from build123d import *

# Parameters (mm, degrees)
SKETCH1_R                                       = 15.875
SKETCH1_R_2                                     = 6.9
BOSS_EXTRUDE1_DEPTH                             = 1
CSK_FOR_M2_FLAT_HEAD_MACHINE_SCREW1_D           = 1
CSK_FOR_M2_FLAT_HEAD_MACHINE_SCREW1_CSINK_D     = 1.6
CSK_FOR_M2_FLAT_HEAD_MACHINE_SCREW1_CSINK_ANGLE = 100
CUT_EXTRUDE1_DEPTH                              = 23.472900347
CUT_EXTRUDE1_DEPTH_BACK                         = 23.472900347
SKETCH4_R                                       = 0.25
SKETCH4_R_2                                     = 1


with BuildPart() as part:
    # Sketch1 → Boss-Extrude1 (new body)
    with BuildSketch(Plane(origin=(0, 0, 0), x_dir=(1, 0, 0), z_dir=(0, 1, 0))):
        with Locations(Location((0, 0, 0), (0, 0, 270))):
            Circle(SKETCH1_R)
        with Locations(Location((0, 0, 0), (0, 0, 270))):
            Circle(SKETCH1_R_2, mode=Mode.SUBTRACT)
    extrude(amount=BOSS_EXTRUDE1_DEPTH)

    # CSK for M2 Flat Head Machine Screw1 (through all)
    with Locations(Plane(origin=(0, 0, 0), x_dir=(-1, 0, 0), z_dir=(0, -1, 0))):
        with Locations((0, -14.29), (-14.29, 0), (0, 14.29), (14.29, 0)):
            CounterSinkHole(CSK_FOR_M2_FLAT_HEAD_MACHINE_SCREW1_D / 2, CSK_FOR_M2_FLAT_HEAD_MACHINE_SCREW1_CSINK_D / 2, counter_sink_angle=CSK_FOR_M2_FLAT_HEAD_MACHINE_SCREW1_CSINK_ANGLE)

    # Sketch4 → Cut-Extrude1 (cut, two sides: drawn at the far end of the back side and taken through both)
    with BuildSketch(Plane(origin=(0, 1, 0), x_dir=(1, 0, 0), z_dir=(0, 1, 0)).offset(-CUT_EXTRUDE1_DEPTH_BACK)):
        with Locations(Location((0, 10.25, 0), (0, 0, 270))):
            Circle(SKETCH4_R)
        with Locations(Location((-7.778174593, -7.778174593, 0), (0, 0, 270))):
            Circle(SKETCH4_R_2)
    extrude(amount=CUT_EXTRUDE1_DEPTH + CUT_EXTRUDE1_DEPTH_BACK, mode=Mode.SUBTRACT)


solid = part.part
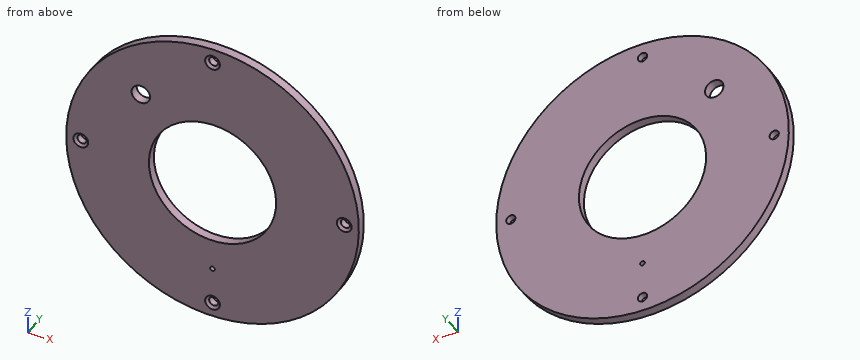
The listing builds one solid part. Answer for the finished solid, in the listing's coordinates (mm). Coordinates: 2 decimals unless noted, no trailing zeros. Write each loop counter-clockwise with the first axis right and the second up, starting at its lowest first coordinate (ties: lowest second). Pieces come first, ordered by that corner, then holes. Notation, with made-up numbers: (8, 46.5) - (51, 46.5) arc R24 ccw to (51, 75.5) - close; hole circle Ø9 at (87.5, 28.25). An arc over 180 degrees is marked (long way). Return JSON: item names as keys, results as strings.
1. The part is cut by section A-A on z = 0. Determine the outline of the cut face in (x, y) (3 decimals).
Final values:
{"outline": "(-15.875, 0) - (-15.09, 0) - (-14.79, 0.252) - (-14.79, 1) - (-15.875, 1) - close; (-13.79, 0.252) - (-13.49, 0) - (-6.9, 0) - (-6.9, 1) - (-13.79, 1) - close; (6.9, 0) - (13.49, 0) - (13.79, 0.252) - (13.79, 1) - (6.9, 1) - close; (14.79, 0.252) - (15.09, 0) - (15.875, 0) - (15.875, 1) - (14.79, 1) - close"}
2. The part is cut by section D-D on z = -14.29. Determine the outline of the cut face in (x, y), then the cut area to 3 significant figures.
Final values:
{"outline": "(-6.91, 0) - (-0.8, 0) - (-0.5, 0.25) - (-0.5, 1) - (-6.91, 1) - close; (0.5, 0.25) - (0.8, 0) - (6.91, 0) - (6.91, 1) - (0.5, 1) - close", "area": "12.8 mm^2"}
3. Consider line 1 along Z through (x, y) = (1.5, 0.6); line 2 along Z through (x, y) = (-7, 0.15); line 3 along X through (y, z) = (0.6, -5.5). Determine where each line is inside the solid, lowest interval first.
Final values:
{"line 1": "-15.8 to -6.73, 6.73 to 15.8", "line 2": "-14.25 to 7.15, 8.41 to 14.25", "line 3": "-14.89 to -4.17, 4.17 to 14.89"}
4. The part is cut by section C-C on y = 0.85. Determine the outline of the cut face in (x, z) (3 decimals), then the cut area to 3 significant figures.
Final values:
{"outline": "circle Ø31.75 at (0, 0); hole circle Ø1 at (-14.29, 0); hole circle Ø2 at (-7.778, 7.778); hole circle Ø13.8 at (0, 0); hole circle Ø1 at (0, -14.29); hole circle Ø1 at (0, 14.29); hole circle Ø0.5 at (0, -10.25); hole circle Ø1 at (14.29, 0)", "area": "636 mm^2"}
5. The part is cut by section B-B on x = -14.29. Determine the outline of the cut face in (y, z).
Final values:
{"outline": "(0, -6.91) - (1, -6.91) - (1, -0.5) - (0.25, -0.5) - (0, -0.8) - close; (0, 0.8) - (0.25, 0.5) - (1, 0.5) - (1, 6.91) - (0, 6.91) - close"}
